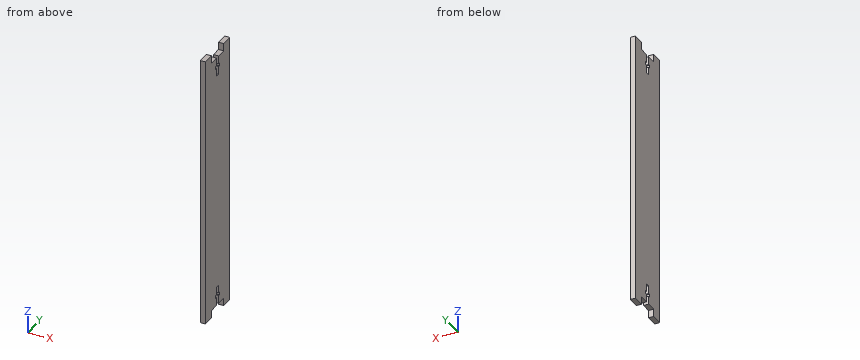
Autodesk Inventor part; units mm, degrees
ref_plane "YZ Plane" through (0, 0, 0) normal (1, 0, 0) x (0, 1, 0)
ref_plane "XZ Plane" through (0, 0, 0) normal (0, 1, 0) x (-1, 0, 0)
ref_plane "XY Plane" through (0, 0, 0) normal (0, 0, 1) x (1, 0, 0)
sketch "Эскиз1" plane through (0, 0, 0) normal (0, 0, 1) x (1, 0, 0)
  line L0 (-2, 18) -> (2, 18)
  line L1 (2, -18) -> (-2, -18)
  line L2 (-2, 18) -> (2, -18) construction
  line L3 (2, 18) -> (-2, -18) construction
  line L4 (-2, 9) -> (2, 9)
  line L5 (2, -9) -> (-2, -9)
  line L6 (-2, 9) -> (2, -9) construction
  line L7 (2, 9) -> (-2, -9) construction
  line L8 (-2, -18) -> (-2, -9)
  line L9 (-2, 9) -> (-2, 18)
  line L10 (2, 18) -> (2, 9)
  line L11 (2, -9) -> (2, -18)
  point P0 (0, 0)
  dimension "d4" = 36
  dimension "d5" = 4
extrude "Выдавливание1" add sketch "Эскиз1" along normal blind 6
sketch "Эскиз2" plane through (0, 0, 6) normal (0, 0, 1) x (1, 0, 0)
  line L0 (-2, -18) -> (2, -18)
  line L1 (2, 18) -> (-2, 18)
  line L2 (-2, -18) -> (2, -18)
  line L3 (2, -18) -> (2, 18)
  line L4 (2, 18) -> (-2, 18)
  line L5 (-2, 18) -> (-2, -18)
  point P0 (0, 0)
extrude "Выдавливание2" add sketch "Эскиз2" along normal blind 201.8
sketch "Эскиз4" plane through (0, 0, 207.8) normal (0, 0, 1) x (1, 0, 0)
  line L0 (2, 18) -> (-2, 18)
  line L1 (-2, -18) -> (2, -18)
  line L2 (-2, 18) -> (2, 18)
  line L3 (2, -18) -> (-2, -18)
  line L4 (-2, 9) -> (-2, -9)
  line L5 (2, 9) -> (-2, 9)
  line L6 (-2, -9) -> (2, -9)
  line L7 (2, 9) -> (-2, -9) construction
  line L8 (-2, 9) -> (2, -9) construction
  line L9 (2, 18) -> (2, 9)
  line L10 (2, -9) -> (2, -18)
  line L11 (-2, -18) -> (-2, -9)
  line L12 (-2, 9) -> (-2, 18)
  point P0 (0, 0)
extrude "Выдавливание3" add sketch "Эскиз4" along normal blind 6
sketch "Эскиз5" plane through (-2, -18, 0) normal (-1, 0, 0) x (0, 0, 1)
  line L0 (106.9, -127.9343) -> (106.9, 327.3325) construction
  line L1 (207.8, 27) -> (207.8, 9)
  line L2 (192.8, 19.575) -> (192.8, 16.425)
  line L3 (207.8, 16.425) -> (207.8, 19.575)
  line L4 (207.8, 19.575) -> (192.8, 16.425) construction
  line L5 (192.8, 19.575) -> (207.8, 16.425) construction
  line L6 (201.45, 15.25) -> (199.15, 15.25)
  line L7 (199.15, 20.75) -> (201.45, 20.75)
  line L8 (201.45, 15.25) -> (199.15, 20.75) construction
  line L9 (199.15, 15.25) -> (201.45, 20.75) construction
  line L10 (201.45, 20.75) -> (201.45, 19.575)
  line L11 (201.45, 16.425) -> (201.45, 15.25)
  line L12 (207.8, 19.575) -> (201.45, 19.575)
  line L13 (199.15, 19.575) -> (192.8, 19.575)
  line L14 (192.8, 16.425) -> (199.15, 16.425)
  line L15 (201.45, 16.425) -> (207.8, 16.425)
  line L16 (199.15, 15.25) -> (199.15, 16.425)
  line L17 (199.15, 19.575) -> (199.15, 20.75)
  line L18 (6, 27) -> (6, 9)
  line L19 (21, 19.575) -> (21, 16.425)
  line L20 (6, 16.425) -> (6, 19.575)
  line L21 (6, 19.575) -> (21, 16.425) construction
  line L22 (21, 19.575) -> (6, 16.425) construction
  line L23 (12.35, 15.25) -> (14.65, 15.25)
  line L24 (14.65, 20.75) -> (12.35, 20.75)
  line L25 (12.35, 15.25) -> (14.65, 20.75) construction
  line L26 (14.65, 15.25) -> (12.35, 20.75) construction
  line L27 (12.35, 20.75) -> (12.35, 19.575)
  line L28 (12.35, 16.425) -> (12.35, 15.25)
  line L29 (6, 19.575) -> (12.35, 19.575)
  line L30 (14.65, 19.575) -> (21, 19.575)
  line L31 (21, 16.425) -> (14.65, 16.425)
  line L32 (12.35, 16.425) -> (6, 16.425)
  line L33 (14.65, 15.25) -> (14.65, 16.425)
  line L34 (14.65, 19.575) -> (14.65, 20.75)
  point P0 (6, 27)
  point P1 (6, 9)
  point P2 (200.3, 18)
  point P3 (207.8, 18)
  point P4 (13.5, 18)
  point P5 (6, 18)
  point P6 (207.8, 19.575)
  dimension "d25" = 15
  dimension "d26" = 3.15
  dimension "d27" = 2.3
  dimension "d28" = 5.5
extrude "Выдавливание4" cut sketch "Эскиз5" against normal blind 6
properties part number "ребро"
Verification items for the finished model (mm, model axes). Give positions to 0.01 mm unless a question says otherwise; leave off trailing zeros. Order: outer loops, then holes, each group sorted by start corner. A loop starts at its lowest first (then second) coordinate and runs counter-clockwise, first axis right, second up. Notation, with made-up numbers: M 80,68 L 102,68 A7 ccw 102,76 Z; hole C 63.5,-9 d10. An arc over 180 degrees is marked long. Answer as a JSON object with one key per item and string values. Group by question number.
1) Cross-section at A-A (z = 18.5). Enter the section's corners in (x, y) (3 decimals).
2) Depth check by flat-ended pin: pin 1 Ø0.6 at (x, y) = (0.5, 2.5) entering from -Z; pin 2 Ø0.9 at (x, y) = (-0.5, -2) entering from +Z. Enter the tip coordinate at first touch or a pass-through.
3) Scan lines: line 1 along Y through (x, z) = (0.15, 204) (3 decimals); line 2 along Z through (x, y) = (0.7, 1.5); line 3 along Z through (x, y) = (0.05, 8.5). Record each from-to range of solid material in increasing order. Write a range as [from, to].
Result sheet:
{
 "1": {"outline": "M -2,-18 L 2,-18 L 2,-1.575 L -2,-1.575 Z; M -2,1.575 L 2,1.575 L 2,18 L -2,18 Z"},
 "2": {"pin 1": "stops at z = 6", "pin 2": "stops at z = 207.8"},
 "3": {"line 1": "y = [-18, -1.575], [1.575, 18]", "line 2": "z = [21, 192.8]", "line 3": "z = [6, 207.8]"}
}
